Geometry: final body of the model. Coordinates: model frame, mm. A direction names the side the tool comes from. Give positions to 0.01 mm unless a question says otherwise; leave off trailing zeros. Write each loop counter-clockwise with the first axis right and the second up, starting at its lowest first coordinate (ties: lowest second). Pieces come first, ordered by that corner, then holes.
Q1. Draft query along Z for faces 4 (the face through (-0.89, 3.04, -0.84)), 5 (the face through (-35.11, 3.04, -29.46)), 6 (the face through (-8, 2, -15)), 7 (the face through (-18, 0, -15)). Return one class per face: pulls with the +Z half, pulls with the -Z half, needs draft (parallel to the pull), parting line crosses it, or undercut.
Q2. Cut plane B-B on y = 2.5. Return the cut outline in (x, z), plus the area to 3 significant figures.
Q3. Cut plane A-A on x = -4. Return the cut outline in (y, z), plus the area to 3 significant figures.
Q4. Reachability of faces 1 (the face through (-15, 2, -15)), 2 (the face through (-30.85, 3.46, -1.78)), 3 (the face through (0, 3, -15)) from +Z, -Z, +X, -X, +Y, -Y: full face, straight path, thin tool, end or side. Return the list, or none.
Q5. Cut plane C-C on z = -25.75. Return the cut outline in (x, y).
Q6. Pin query (flat end, axial travel): pin 1 (1.8 mm diameter, centred on x = -5, z = -3.5, fed in from +Y); pin 2 (2 mm diameter, centred on x = -11.5, z = -20, fed in from -Y); pin 3 (2.5 mm diameter, centred on x = -32, z = -25.75, fed in from -Y); pin 4 (2 mm diameter, centred on x = -13.5, z = -26.5, fed in from -Y). Return the tip coordinate at first contact, or that it passes through.
Q7. Cut plane D-D on z = -10.5. Return the cut outline in (x, y), plus the area to 3 significant figures.
Q8. Line query: L1, parallel to X at y = 3.7, z = -25.75; L2, parallel to Z at x = -32, y = 0.35; L3, parallel to Z at x = -32, y = 4.8. Output: solid intervals per line, ascending.
Autodesk Inventor part; units mm, degrees
ref_plane "РабПлоскость3" through (-8, 0, 0) normal (1, 0, 0) x (0, 0, -1)
ref_plane "YZ Plane" through (0, 0, 0) normal (1, 0, 0) x (0, 1, 0)
ref_plane "XZ Plane" through (0, 0, 0) normal (0, 1, 0) x (-1, 0, 0)
sketch "Эскиз1" plane through (0, 0, 0) normal (0, 1, 0) x (-1, 0, 0)
  line L0 (0, 0) -> (36, 0)
  line L1 (36, 0) -> (36, -30.3)
  line L2 (36, -30.3) -> (0, -30.3)
  line L3 (0, -30.3) -> (0, 0)
  dimension "d0" = 36
  dimension "d1" = 30.3
extrude "Выдавливание1" add sketch "Эскиз1" along normal blind 6
sketch "Эскиз2" plane through (0, 6, 0) normal (0, 1, 0) x (1, 0, 0)
  line L0 (-36, 30.3) -> (-36, 0)
  line L1 (-36, 0) -> (0, 0)
  line L2 (-18, 0) -> (-18, 30.3)
  line L3 (0, 30.3) -> (-36, 30.3)
  line L4 (-36, 15.15) -> (0, 15.15)
  line L5 (0, 0) -> (0, 30.3)
  point P0 (-32, 4.55)
  point P1 (-32, 25.75)
  point P2 (-4, 4.55)
  point P3 (-4, 25.75)
  point P4 (-32, 4.55)
  dimension "d52" = 14
  dimension "d53" = 10.6
hole "Отверстие1" at (-32, 6, -4.55) at (-32, 6, -25.75) at (-4, 6, -25.75) at (-4, 6, -4.55) direction (0, -1, 0) diameter 3.2 end through all counterbore diameter 6 counterbore depth 5
sketch "Эскиз4" plane through (0, 0, -2.95) normal (1, 0, 0) x (0, 0, -1)
  line L0 (12.2, 0) -> (12.2, -13.5)
  circle A0 centre (12.2, -13.5) radius 18.5
  line L1 (-2.95, 3) -> (27.35, 3)
  line L2 (-2.95, 0) -> (-2.95, 6)
  line L3 (27.35, 0) -> (27.35, 6)
  line L4 (-2.95, 0) -> (27.35, 0)
  dimension "d27" = 13.5
  dimension "d38" = 37
ref_plane "РабПлоскость3" through (-8, 0, 0) normal (1, 0, 0) x (0, 0, -1)
ref_plane "РабПлоскость2" through (-18, 0, 0) normal (1, 0, 0) x (0, 0, -1)
extrude "Выдавливание3" cut sketch "Эскиз4" against normal blind 7 from surface at -8 contours A0 L4 | L4 A0 L1 | L1 A0
fillet "Сопряжение3" radius 2.95 4 edges at (-36, 3, 0) (-36, 3, -30.3) (0, 3, 0) (0, 3, -30.3)
equation "\"Радиус_гибки\" = Толщина"
equation "\"Ширина_просечки\" = Толщина"
equation "\"Глубина_просечки\" = 0.5 * Толщина"
equation "\"Размер_просечки\" = 4 * Толщина"
equation "\"Мин_остаток\" = 2 * Толщина"
equation "\"Радиус_перехода\" = Радиус_гибки"
equation "\"Радиус_Якоби\" = Толщина"
equation "\"Размер_зазора\" = Толщина"
properties part number "Крепление двигателя2"
Data:
1. face 4: pulls with the +Z half
1. face 5: pulls with the -Z half
1. face 6: undercut
1. face 7: needs draft
2. outline: (-36, -27.35) arc R2.95 ccw to (-33.05, -30.3) - (-2.95, -30.3) arc R2.95 ccw to (0, -27.35) - (0, -2.95) arc R2.95 ccw to (-2.95, 0) - (-33.05, 0) arc R2.95 ccw to (-36, -2.95) - close; hole circle Ø6 at (-32, -25.75); hole circle Ø6 at (-32, -4.55); hole (-15, -24.44) - (-8, -24.44) - (-8, -5.86) - (-15, -5.86) - close; hole circle Ø6 at (-4, -25.75); hole circle Ø6 at (-4, -4.55)
2. area: 840 mm2
3. outline: (0, -30.3) - (6, -30.3) - (6, -28.75) - (1, -28.75) - (1, -27.35) - (0, -27.35) - close; (0, -24.15) - (1, -24.15) - (1, -22.75) - (6, -22.75) - (6, -7.55) - (1, -7.55) - (1, -6.15) - (0, -6.15) - close; (0, -2.95) - (1, -2.95) - (1, -1.55) - (6, -1.55) - (6, 0) - (0, 0) - close
3. area: 115 mm2
4. face 1: -Y
4. face 2: +Y
4. face 3: +Z, -Z, +X, +Y, -Y
5. outline: (-36, 0) - (-33.6, 0) - (-33.6, 1) - (-35, 1) - (-35, 6) - (-36, 6) - close; (-30.4, 0) - (-15, 0) - (-15, 1.66) - (-8, 1.66) - (-8, 0) - (-5.6, 0) - (-5.6, 1) - (-7, 1) - (-7, 6) - (-29, 6) - (-29, 1) - (-30.4, 1) - close; (-2.4, 0) - (0, 0) - (0, 6) - (-1, 6) - (-1, 1) - (-2.4, 1) - close
6. pin 1: stops at y = 1
6. pin 2: stops at y = 4.05
6. pin 3: passes through
6. pin 4: stops at y = 0.27
7. outline: (-36, 0) - (-15, 0) - (-15, 4.41) - (-8, 4.41) - (-8, 0) - (0, 0) - (0, 6) - (-36, 6) - close
7. area: 185 mm2
8. L1: x = -36 to -35, -29 to -7, -1 to 0
8. L2: z = -30.3 to -27.35, -24.15 to -6.15, -2.95 to 0
8. L3: z = -30.3 to -28.75, -22.75 to -7.55, -1.55 to 0
